from build123d import *

# Parameters (mm, degrees)
SKETCH1_W           = 13.2461
SKETCH1_H           = 10.668
SKETCH1_R           = 3.93065
BOSS_EXTRUDE1_DEPTH = 3.175
SKETCH1_2_R         = 3.93065
SKETCH1_2_R_2       = 0.79375
BOSS_EXTRUDE2_DEPTH = 100.711
FILLET1_R           = 4.445


with BuildPart() as part:
    # Sketch1 → Boss-Extrude1 (new body)
    with BuildSketch(Plane.XY):
        with Locations((6.62305, 5.334)):
            Rectangle(SKETCH1_W, SKETCH1_H)
        with Locations((6.62305, 5.334)):
            Circle(SKETCH1_R, mode=Mode.SUBTRACT)
    extrude(amount=BOSS_EXTRUDE1_DEPTH)

    # Sketch1<2> → Boss-Extrude2 (add)
    with BuildSketch(Plane.XY):
        with Locations((6.62305, 5.334)):
            Circle(SKETCH1_2_R)
        with Locations((6.62305, 5.334)):
            Circle(SKETCH1_2_R_2, mode=Mode.SUBTRACT)
    extrude(amount=BOSS_EXTRUDE2_DEPTH)

    # Fillet1
    fillet1_edges = [part.edges().sort_by_distance(p)[0] for p in [
        (0, 0, 1.5875),
        (0, 10.668, 1.5875),
        (13.2461, 10.668, 1.5875),
        (13.2461, 0, 1.5875),
    ]]
    fillet(fillet1_edges, radius=FILLET1_R)


solid = part.part
Read the model definition and answer for the solid it produces. Units are mm, in the model's axes. A direction names the side the tool comes from. Give positions to 0.01 mm unless a question says otherwise; leave off trailing zeros. Write each loop counter-clockwise with the first axis right and the second up, starting at its lowest first coordinate (ties: lowest second). Pieces come first, ordered by that corner, then holes. Notation, with made-up numbers: (86.25, -4) - (138.25, -4) arc R22 ccw to (138.25, 19) - close; hole circle Ø10 at (55, -10.75). An arc over 180 degrees is marked (long way). Answer in a Markdown table with one row per item. Add a question column.
Item 1: Section A-A, the plane y = 2.5 is taken. Write down the section's boundary in (x, z) (3 decimals).
Item 2: Find the intervals of material crossed by L1, parallel to Z at x = 2, y = 6.75 (3 decimals); L2, parallel to Y at x = 6.75, z = 87; L3, parallel to Y at x = 7, z = 30, in increasing order.
Item 3: Flat-ended cylindrical pins translate along their axes: P1, Ø5, axis at x = 2.5, z = 69, coming from the +Y side; P2, Ø6, axis at x = 8, z = 47.5, coming from the +Y side; P3, Ø2, axis at x = 4.5, z = 40, coming from the +Y side. Find the tip coordinate at first contact, or state that the pin passes through.
Item 4: Determine the mould class of faces 3 (the face through (7.38, 5.57, 49.65)), 4 (the face through (0, 5, 2)), 5 (the face through (8.44, 1.85, 51.26)) for opening direction Y: pulls with the +Y half, pulls with the -Y half, needs draft (parallel to the pull), parting line crosses it, or undercut.
Item 5: A tool of negligible diameter and unlimited length cuts with its end or side. For faces 1 (the face through (2, 5, 3.175)), 2 (the face through (7, 0, 2)), from which of +Z, -Z, +X, -X, +Y, -Y can it reach the whole face along a straight path? Write none if from no direction.
Item 6: Section C-C, the plane x = 1.75 is taken. Write down the section's boundary in (y, z) (3 decimals), and give its area (3 significant figures).
Item 7: Section B-B, the plane z = 48 is taken. Write down the section's boundary in (x, y).
Recorded:
| question | item | result |
|---|---|---|
| 1 | outline | (0.448, 0) - (12.798, 0) - (12.798, 3.175) - (9.347, 3.175) - (9.347, 100.711) - (3.899, 100.711) - (3.899, 3.175) - (0.448, 3.175) - close |
| 2 | L1 | z = 0 to 3.175 |
| 2 | L2 | y = 1.41 to 4.55, 6.12 to 9.26 |
| 2 | L3 | y = 1.42 to 4.64, 6.03 to 9.25 |
| 3 | P1 | stops at y = 8.91 |
| 3 | P2 | stops at y = 9.26 |
| 3 | P3 | stops at y = 9.1 |
| 4 | face 3 | undercut |
| 4 | face 4 | needs draft |
| 4 | face 5 | parting line crosses it |
| 5 | face 1 | +Z |
| 5 | face 2 | +Z, -Z, +X, -X, -Y |
| 6 | outline | (0.91, 0) - (9.758, 0) - (9.758, 3.175) - (0.91, 3.175) - close |
| 6 | area | 28.1 mm2 |
| 7 | outline | circle Ø7.86 at (6.62, 5.33); hole circle Ø1.59 at (6.62, 5.33) |
